Input: part model. Units: mm. Frame: model coordinates. A direction names the side the tool comes from. Give positions to 0.01 mm unless a question says otherwise; leave off trailing zeros. Loops run counter-clockwise (first coordinate to the right, second up) from the corner with the lowest first, then second, coordinate; pieces in that order, holes last. Notation, with made-up numbers: (65.25, 58.25) -> (76.25, 58.25) arc R12 cw to (76.25, 66.25) -> close; hole circle Ø6 at (35, -39.5). An arc over 180 degrees is marked (long way). Answer in a Markdown table with one row per item. Add a question column.
```python
from build123d import *

# Parameters (mm, degrees)
SKETCH1_W           = 100
SKETCH1_H           = 247
SKETCH1_R           = 2.625
SKETCH1_R_2         = 4
BOSS_EXTRUDE1_DEPTH = 7
SKETCH2_R           = 11.025
CUT_EXTRUDE1_DEPTH  = 3
CUT_EXTRUDE2_DEPTH  = 3
SKETCH4_W           = 100
SKETCH4_H           = 80
CUT_EXTRUDE3_DEPTH  = 134.421325132


with BuildPart() as part:
    # Sketch1 → Boss-Extrude1 (new body)
    with BuildSketch(Plane.XY):
        Rectangle(SKETCH1_W, SKETCH1_H)
        with Locations((-42, -34.5)):
            Circle(SKETCH1_R, mode=Mode.SUBTRACT)
        with Locations((42, -34.5)):
            Circle(SKETCH1_R, mode=Mode.SUBTRACT)
        with Locations((-42, -115.5)):
            Circle(SKETCH1_R, mode=Mode.SUBTRACT)
        with Locations((42, -115.5)):
            Circle(SKETCH1_R, mode=Mode.SUBTRACT)
        with Locations((0, 18.5)):
            Circle(SKETCH1_R_2, mode=Mode.SUBTRACT)
        with Locations((42, 115.5)):
            Circle(SKETCH1_R, mode=Mode.SUBTRACT)
        with Locations((-42, 115.5)):
            Circle(SKETCH1_R, mode=Mode.SUBTRACT)
        with BuildLine():
            Line((-19.05, -80.5), (-19.05, -86.5))
            ThreePointArc((-19.05, -86.5), (0, -105.55), (19.05, -86.5))
            Line((19.05, -86.5), (19.05, -80.5))
            ThreePointArc((19.05, -80.5), (0, -61.45), (-19.05, -80.5))
        make_face(mode=Mode.SUBTRACT)
        with BuildLine():
            Line((-22.25, -55), (-22.25, -65))
            ThreePointArc((-22.25, -65), (-23.5, -66.25), (-24.75, -65))
            Line((-24.75, -65), (-24.75, -55))
            ThreePointArc((-24.75, -55), (-23.5, -53.75), (-22.25, -55))
        make_face(mode=Mode.SUBTRACT)
        with BuildLine():
            Line((22.25, -55), (22.25, -65))
            ThreePointArc((22.25, -65), (23.5, -66.25), (24.75, -65))
            Line((24.75, -65), (24.75, -55))
            ThreePointArc((24.75, -55), (23.5, -53.75), (22.25, -55))
        make_face(mode=Mode.SUBTRACT)
        with BuildLine():
            Line((22.25, -112), (22.25, -102))
            ThreePointArc((22.25, -102), (23.5, -100.75), (24.75, -102))
            Line((24.75, -102), (24.75, -112))
            ThreePointArc((24.75, -112), (23.5, -113.25), (22.25, -112))
        make_face(mode=Mode.SUBTRACT)
        with BuildLine():
            Line((-22.25, -112), (-22.25, -102))
            ThreePointArc((-22.25, -102), (-23.5, -100.75), (-24.75, -102))
            Line((-24.75, -102), (-24.75, -112))
            ThreePointArc((-24.75, -112), (-23.5, -113.25), (-22.25, -112))
        make_face(mode=Mode.SUBTRACT)
    extrude(amount=BOSS_EXTRUDE1_DEPTH)

    # Sketch2 → Cut-Extrude1 (cut)
    with BuildSketch(Plane.XY.offset(7)):
        with Locations((0, 18.5)):
            Circle(SKETCH2_R)
    extrude(amount=-CUT_EXTRUDE1_DEPTH, mode=Mode.SUBTRACT)

    # Sketch3 → Cut-Extrude2 (cut)
    with BuildSketch(Plane.XY):
        with BuildLine():
            Line((-26.5, -65), (-26.5, -55))
            ThreePointArc((-26.5, -55), (-23.5, -52), (-20.5, -55))
            Line((-20.5, -55), (-20.5, -65))
            ThreePointArc((-20.5, -65), (-23.5, -68), (-26.5, -65))
        make_face()
        with BuildLine():
            Line((20.5, -65), (20.5, -55))
            ThreePointArc((20.5, -55), (23.5, -52), (26.5, -55))
            Line((26.5, -55), (26.5, -65))
            ThreePointArc((26.5, -65), (23.5, -68), (20.5, -65))
        make_face()
        with BuildLine():
            Line((-26.5, -112), (-26.5, -102))
            ThreePointArc((-26.5, -102), (-23.5, -99), (-20.5, -102))
            Line((-20.5, -102), (-20.5, -112))
            ThreePointArc((-20.5, -112), (-23.5, -115), (-26.5, -112))
        make_face()
        with BuildLine():
            Line((20.5, -112), (20.5, -102))
            ThreePointArc((20.5, -102), (23.5, -99), (26.5, -102))
            Line((26.5, -102), (26.5, -112))
            ThreePointArc((26.5, -112), (23.5, -115), (20.5, -112))
        make_face()
    extrude(amount=CUT_EXTRUDE2_DEPTH, mode=Mode.SUBTRACT)

    # Sketch4 → Cut-Extrude3 (cut, through all)
    with BuildSketch(Plane.XY.offset(7)):
        with Locations((0, 83.5)):
            Rectangle(SKETCH4_W, SKETCH4_H)
    extrude(amount=-CUT_EXTRUDE3_DEPTH, mode=Mode.SUBTRACT)


solid = part.part
```
1) Pull-direction query (Y, two-part tool) for faces 1 (the face through (-1, 43.5, 4)), 2 (the face through (23.4, -52, 1.5)), 3 (the face through (-1, -39, 0)), 4 (the face through (-22.25, -60, 5)); classes: +Y half, -Y half, draft (parallel to the pull), parting line (faces both ways), or undercut.
2) Reachability of faces 5 (the face through (24.75, -107, 5)), 6 (the face through (5, 19, 4)), 7 (the face through (20.5, -60, 1)) from +Z, -Z, +X, -X, +Y, -Y: full face, straight path, thin tool, end or side. Return the list, or none.
3) Material intervals for line 1 along Y through (x, z) = (42, 5) (3 decimals); line 2 along Y through (x, z) = (0, 4.7) (3 decimals); line 3 along X through (y, z) = (-101.5, 6.75), sorted ascending.
4) Section C-C on x = -42. Output: boundary loops of the cut face in (y, z) (3 decimals), and give its area (3 significant figures).
5) Section B-B on z = 1.75. State how many separate pieces and enclosed holes the cut face has, and give its area (3 significant figures).
6) Pin query (flat end, axial travel): pin 1 (5 mm diameter, centred on x = 24.5, y = -110.5, fed in from -Z); pin 2 (1.8 mm diameter, centred on x = 22.5, y = -60, fed in from -Z); pin 3 (9 mm diameter, centred on x = 0, y = 18.5, fed in from +Z). Return the tip coordinate at first contact, or that it passes through.
7) Section A-A on x = 0. Output: boundary loops of the cut face in (y, z) (3 decimals).
Working result:
| question | item | result |
|---|---|---|
| 1 | face 1 | +Y half |
| 1 | face 2 | undercut |
| 1 | face 3 | draft |
| 1 | face 4 | undercut |
| 2 | face 5 | +Z, -Z |
| 2 | face 6 | +Z |
| 2 | face 7 | -Z |
| 3 | line 1 | y = -123.5 to -118.125, -112.875 to -37.125, -31.875 to 43.5 |
| 3 | line 2 | y = -123.5 to -105.55, -61.45 to 7.475, 29.525 to 43.5 |
| 3 | line 3 | x = -50 to -24.65, -22.35 to -11.74, 11.74 to 22.35, 24.65 to 50 |
| 4 | outline | (-123.5, 0) -> (-118.125, 0) -> (-118.125, 7) -> (-123.5, 7) -> close; (-112.875, 0) -> (-37.125, 0) -> (-37.125, 7) -> (-112.875, 7) -> close; (-31.875, 0) -> (43.5, 0) -> (43.5, 7) -> (-31.875, 7) -> close |
| 4 | area | 1,100 mm2 |
| 5 | separate pieces | 1 |
| 5 | enclosed holes | 10 |
| 5 | area | 14,800 mm2 |
| 6 | pin 1 | stops at z = 0 |
| 6 | pin 2 | stops at z = 3 |
| 6 | pin 3 | stops at z = 4 |
| 7 | outline | (-123.5, 0) -> (-105.55, 0) -> (-105.55, 7) -> (-123.5, 7) -> close; (-61.45, 0) -> (14.5, 0) -> (14.5, 4) -> (7.475, 4) -> (7.475, 7) -> (-61.45, 7) -> close; (22.5, 0) -> (43.5, 0) -> (43.5, 7) -> (29.525, 7) -> (29.525, 4) -> (22.5, 4) -> close |
